Build history of the part. All positions in model axes, mm. Face numbers are marked on the shaded views. A direction names the side the tool comes from. Give positions to 0.01 mm unless a question says otherwise; leave off trailing zeros. Write each loop counter-clockwise with the first axis right and the second up, starting at its lowest first coordinate (ties: lowest second). Pieces come first, ordered by that corner, then holes. Notation, with made-up numbers: M -9.75,69 L 42.25,69 A5 cw 42.25,73 Z; hole C 29,58 d2. An arc over 180 degrees is marked long. One line per item, written item: value. Start each with the question number.
from build123d import *

# Parameters (mm, degrees)
SALIENTE_EXTRUIR1_DEPTH      = 60
SALIENTE_EXTRUIR1_DEPTH_BACK = 5
CROQUIS1_W                   = 30
CROQUIS1_H                   = 30
CROQUIS2_W                   = 26
CROQUIS2_H                   = 26
CORTAR_EXTRUIR3_DEPTH        = 65
CROQUIS3_W                   = 20
CROQUIS3_H                   = 45
CORTAR_EXTRUIR4_DEPTH        = 2
CROQUIS4_W                   = 26
CROQUIS4_H                   = 26
SALIENTE_EXTRUIR2_DEPTH      = 5
CROQUIS5_R                   = 8.5
CORTAR_EXTRUIR5_DEPTH        = 5


with BuildPart() as part:
    # Croquis1 → Saliente-Extruir1 (new, two sides: drawn at the far end of the back side and taken through both)
    with BuildSketch(Plane(origin=(0, 0, 0), x_dir=(1, 0, 0), z_dir=(0, 1, 0)).offset(-SALIENTE_EXTRUIR1_DEPTH_BACK)):
        Rectangle(CROQUIS1_W, CROQUIS1_H)
    extrude(amount=SALIENTE_EXTRUIR1_DEPTH + SALIENTE_EXTRUIR1_DEPTH_BACK)

    # Croquis2 → Cortar-Extruir3 (cut)
    with BuildSketch(Plane(origin=(0, 60, 0), x_dir=(1, 0, 0), z_dir=(0, 1, 0))):
        Rectangle(CROQUIS2_W, CROQUIS2_H)
    extrude(amount=-CORTAR_EXTRUIR3_DEPTH, mode=Mode.SUBTRACT)

    # Croquis3 → Cortar-Extruir4 (cut)
    with BuildSketch(Plane(origin=(15, 0, 0), x_dir=(0, 0, -1), z_dir=(1, 0, 0))):
        with Locations((3, 32.5)):
            Rectangle(CROQUIS3_W, CROQUIS3_H)
    extrude(amount=-CORTAR_EXTRUIR4_DEPTH, mode=Mode.SUBTRACT)

    # Croquis4 → Saliente-Extruir2 (add)
    with BuildSketch(Plane.XZ.offset(5)):
        Rectangle(CROQUIS4_W, CROQUIS4_H)
    extrude(amount=-SALIENTE_EXTRUIR2_DEPTH)

    # Croquis5 → Cortar-Extruir5 (cut)
    with BuildSketch(Plane.XZ.offset(5)):
        with Locations(Location((0, 0, 0), (0, 0, 270))):
            Circle(CROQUIS5_R)
    extrude(amount=-CORTAR_EXTRUIR5_DEPTH, mode=Mode.SUBTRACT)


solid = part.part
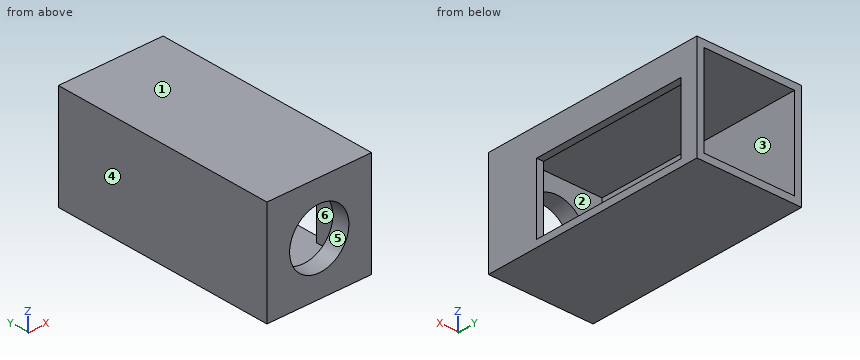
1) Band-saw the part on C-C (y = 28.5). List the corners of the cut face in (x, z), then the cut area to 3 significant figures.
2) Band-saw the part on A-A (x = -5.75). List the corners of the cut face in (y, z), then the cut area to 3 significant figures.
3) Tool access for the marked faces 5 and 6: list every direction of +Z, -Z, +X, -X, +Y, -Y with a clear straight run to the whole face (end or side of a thin tool).
4) Band-saw the part on B-B (z = 0). List the corners of the cut face in (x, y), then the cut area to 3 significant figures.
5) Mould opens along X. For the marked faces 1, 2, 3 and 4 say: released by +X, released by -X, zero draft, split by the parting line, or undercut.
6) Probe line 1 along Y through (x, z) = (13.5, -4.5); line 2 along Z through (x, y) = (10.5, 28.5); line 3 along X through (y, z) = (-1.45, 0). List the from-to ranges inside material, lowest first. Write a range as from..to.
7) Band-saw the part on D-D (x = 0). List the corners of the cut face in (y, z).
Model answer:
1. outline: M -15,-15 L 15,-15 L 15,-13 L -13,-13 L -13,13 L 13,13 L 13,7 L 15,7 L 15,15 L -15,15 Z
1. area: 184 mm²
2. outline: M -5,-15 L 60,-15 L 60,-13 L 0,-13 L 0,-6.26 L -5,-6.26 Z; M -5,6.26 L 0,6.26 L 0,13 L 60,13 L 60,15 L -5,15 Z
2. area: 327 mm²
3. face 5: +Y, -Y
3. face 6: +Y
4. outline: M -15,-5 L -8.5,-5 L -8.5,0 L -13,0 L -13,60 L -15,60 Z; M 8.5,-5 L 15,-5 L 15,10 L 13,10 L 13,0 L 8.5,0 Z; M 13,55 L 15,55 L 15,60 L 13,60 Z
4. area: 215 mm²
5. face 1: zero draft
5. face 2: undercut
5. face 3: undercut
5. face 4: released by -X
6. line 1: y = -5..10, 55..60
6. line 2: z = -15..-13, 13..15
6. line 3: x = -15..-8.5, 8.5..15
7. outline: M -5,-15 L 60,-15 L 60,-13 L 0,-13 L 0,-8.5 L -5,-8.5 Z; M -5,8.5 L 0,8.5 L 0,13 L 60,13 L 60,15 L -5,15 Z
